Geometry: final body of the model. Coordinates: model frame, mm. Face numbers are marked on the shaded views. A direction names the side the tool comes from. Round coordinates to 2 decimals unless told otherwise and drop trailing zeros. Write each loop counter-clockwise with the first axis right and the second up, starting at its lowest first coordinate (ties: lowest second). Pieces come first, ordered by that corner, then holes. Notation, with made-up numbers: M 71.5,76.5 L 127.5,76.5 A16 ccw 127.5,104.5 Z; hole C 51.5,49.25 d8. An arc over 180 degrees is marked long. Put each result on its own line as item: value. Start each with the question number.
```python
from build123d import *

# Parameters (mm, degrees)
SKETCH1_W           = 12.25
SKETCH1_H           = 42.3
BOSS_EXTRUDE1_DEPTH = 6.125
SKETCH2_R           = 1.825
SKETCH2_R_2         = 2.5
CUT_EXTRUDE1_DEPTH  = 23.855059615
CUT_EXTRUDE2_DEPTH  = 23.855059615
SKETCH4_R           = 11.5
CUT_EXTRUDE3_DEPTH  = 2.625
BOSS_EXTRUDE2_START = 0.5
SKETCH5_R           = 4.8
SKETCH5_R_2         = 2.5
BOSS_EXTRUDE2_DEPTH = 0.5
BOSS_EXTRUDE3_START = 2.125
SKETCH6_R           = 3.8
SKETCH6_R_2         = 2.5
BOSS_EXTRUDE3_DEPTH = 2.125
BOSS_EXTRUDE4_REACH = 27.197
CUT_EXTRUDE4_DEPTH  = 26.19723458


with BuildPart() as part:
    # Sketch1 → Boss-Extrude1 (new body)
    with BuildSketch(Plane.XY):
        Rectangle(SKETCH1_W, SKETCH1_H)
    extrude(amount=BOSS_EXTRUDE1_DEPTH)

    # Sketch2 → Cut-Extrude1 (cut, through all)
    with BuildSketch(Plane.XY.offset(6.125)):
        with Locations((0.475, 15.5)):
            Circle(SKETCH2_R)
        with Locations((0.475, 0)):
            Circle(SKETCH2_R_2)
    extrude(amount=-CUT_EXTRUDE1_DEPTH, mode=Mode.SUBTRACT)

    # Sketch3 → Cut-Extrude2 (cut, through all)
    with BuildSketch(Plane.XY.offset(6.125)):
        with BuildLine():
            Line((-6.125, -21.15), (-1.151863079, -21.15))
            ThreePointArc((-1.151863079, -21.15), (-2.238128282, -12.336341525), (-6.125, -4.351807973))
            Line((-6.125, -4.351807973), (-6.125, -21.15))
        make_face()
        with BuildLine():
            Line((6.125, 21.15), (1.764842259, 21.15))
            ThreePointArc((1.764842259, 21.15), (4.069800152, 19.094796032), (6.125, 16.789834467))
            Line((6.125, 16.789834467), (6.125, 21.15))
        make_face()
        with BuildLine():
            Line((6.125, -21.15), (1.757457575, -21.15))
            ThreePointArc((1.757457575, -21.15), (4.066466825, -19.092268783), (6.125, -16.783974467))
            Line((6.125, -16.783974467), (6.125, -21.15))
        make_face()
    extrude(amount=-CUT_EXTRUDE2_DEPTH, mode=Mode.SUBTRACT)

    # Sketch4 → Cut-Extrude3 (cut)
    with BuildSketch(Plane.XY.offset(6.125)):
        with Locations((0.475, 0)):
            Circle(SKETCH4_R)
    extrude(amount=-CUT_EXTRUDE3_DEPTH, mode=Mode.SUBTRACT)

    # Sketch5 → Boss-Extrude2 (add)
    with BuildSketch(Plane.XY.offset(3.5).offset(BOSS_EXTRUDE2_START)):
        with Locations((0.475, 0)):
            Circle(SKETCH5_R)
        with Locations((0.475, 0)):
            Circle(SKETCH5_R_2, mode=Mode.SUBTRACT)
    extrude(amount=-BOSS_EXTRUDE2_DEPTH)

    # Sketch6 → Boss-Extrude3 (add)
    with BuildSketch(Plane.XY.offset(4).offset(BOSS_EXTRUDE3_START)):
        with Locations((0.475, 0)):
            Circle(SKETCH6_R)
        with Locations((0.475, 0)):
            Circle(SKETCH6_R_2, mode=Mode.SUBTRACT)
    extrude(amount=-BOSS_EXTRUDE3_DEPTH)

    # Sketch7 → Boss-Extrude4 (add, up to next)
    with BuildSketch(Plane(origin=(6.125, 0, 0), x_dir=(0, 0, -1), z_dir=(1, 0, 0)), mode=Mode.PRIVATE) as boss_extrude4_sk1:
        with BuildLine():
            Line((-6.125, -13.462065527), (-6.125, -20.957897703))
            ThreePointArc((-6.125, -20.957897703), (-2.25, -17.209981615), (-6.125, -13.462065527))
        make_face()
    boss_extrude4_tool1 = extrude(boss_extrude4_sk1.sketch, amount=-BOSS_EXTRUDE4_REACH, mode=Mode.PRIVATE) - part.part
    add(boss_extrude4_tool1.solids().sort_by_distance((6.125, -17.209982, 4.47578))[0])

    # Sketch8 → Cut-Extrude4 (cut, through all)
    with BuildSketch(Plane(origin=(6.125, 0, 0), x_dir=(0, 0, -1), z_dir=(1, 0, 0))):
        with BuildLine():
            Line((-7.8, -17.973571615), (-7.8, -16.459481615))
            ThreePointArc((-7.8, -16.459481615), (-6, -14.659481615), (-4.2, -16.459481615))
            Line((-4.2, -16.459481615), (-4.2, -17.973571615))
            ThreePointArc((-4.2, -17.973571615), (-6, -19.773571615), (-7.8, -17.973571615))
        make_face()
    extrude(amount=-CUT_EXTRUDE4_DEPTH, mode=Mode.SUBTRACT)


solid = part.part
```
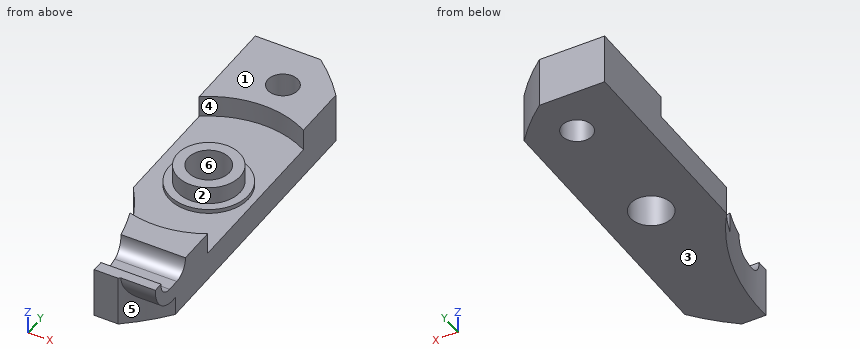
1) First-contact query: pin 1 (1 mm diameter, centred on x = 1.5, y = -16, fed in from +Z); pin 2 (0.5 mm diameter, centred on x = 2.5, y = -17, fed in from +Z). Flat tips, straight axial feed; report the tip coordinate or a pass-through.
2) Draft query along Y for the marked faces 3, 4, 5 and 6. Return one class per face: +Y half, -Y half, draft (parallel to the pull), parting line (faces both ways), or undercut.
3) Section B-B, the plane z = 1.25. Output: boundary loops of the cut face in (x, y) (3 decimals).
4) Ray query, probe 1 along Y at (x, z) = (0.75, 0.5); probe 2 along Y at (x, z) = (1, 5); probe 3 along Y at (x, z) = (1.5, 5.5). Return the intervals inside material, ascending.
5) Section A-A, the plane y = 0. Output: boundary loops of the cut face in (x, z) (3 decimals), and give its area (3 significant figures).
6) Section D-D, the plane x = -0.5. Output: boundary loops of the cut face in (y, z) (3 decimals), and give its area (3 significant figures).
7) Section C-C, the plane z = 4.75. Output: boundary loops of the cut face in (x, y) (3 decimals).
8) Access query for the marked faces 1 and 2. Directions: +Z, -Z, +X, -X, +Y, -Y. A direction counts if a zero-diameter tool reaches every point of the face in a straight line with its end or side. Return the directions, or none.
Solved:
1. pin 1: stops at z = 4.48
1. pin 2: stops at z = 4.2
2. face 3: draft
2. face 4: undercut
2. face 5: -Y half
2. face 6: undercut
3. outline: M -6.125,-4.352 A27 cw -1.152,-21.15 L 1.757,-21.15 A27 ccw 6.125,-16.784 L 6.125,16.79 A27 ccw 1.765,21.15 L -6.125,21.15 Z; hole C 0.475,0 d5; hole C 0.475,15.5 d3.65
4. probe 1: y = -21.15 to -2.48, 2.48 to 13.7, 17.3 to 21.15
4. probe 2: y = -21.15 to -19.47, -14.96 to -11.49, -3.76 to -2.44, 2.44 to 3.76, 11.49 to 13.75, 17.25 to 21.15
4. probe 3: y = -21.15 to -19.7, -14.73 to -11.45, -3.66 to -2.28, 2.28 to 3.66, 11.45 to 13.99, 17.01 to 21.15
5. outline: M -6.125,0 L -2.025,0 L -2.025,6.125 L -3.325,6.125 L -3.325,4 L -4.325,4 L -4.325,3.5 L -6.125,3.5 Z; M 2.975,0 L 6.125,0 L 6.125,3.5 L 5.275,3.5 L 5.275,4 L 4.275,4 L 4.275,6.125 L 2.975,6.125 Z
5. area: 33.2 mm2
6. outline: M -21.15,0 L -2.302,0 L -2.302,6.125 L -3.673,6.125 L -3.673,4 L -4.7,4 L -4.7,3.5 L -11.459,3.5 L -11.459,6.125 L -14.664,6.125 A1.8 cw -16.459,4.2 L -17.974,4.2 A1.8 cw -19.769,6.125 L -21.15,6.125 Z; M 2.302,0 L 13.957,0 L 13.957,6.125 L 11.459,6.125 L 11.459,3.5 L 4.7,3.5 L 4.7,4 L 3.673,4 L 3.673,6.125 L 2.302,6.125 Z; M 17.043,0 L 21.15,0 L 21.15,6.125 L 17.043,6.125 Z
6. area: 164 mm2
7. outline: M -6.125,9.418 A11.5 cw 6.125,10.016 L 6.125,16.79 A27 ccw 1.765,21.15 L -6.125,21.15 Z; C 0.475,0 d7.6; M -2.648,-11.068 A27 cw -1.564,-15.164 L 6.125,-15.164 L 6.125,-10.016 A11.5 cw Z; M -1.152,-21.15 L 1.757,-21.15 A27 ccw 2.255,-20.746 L 6.125,-20.746 L 6.125,-19.269 L -1.137,-19.269 A27 cw Z; hole C 0.475,0 d5; hole C 0.475,15.5 d3.65
8. face 1: +Z, +X, -X, +Y, -Y
8. face 2: +Z
